Geometry: final body of the model. Coordinates: model frame, mm. Give positions to 0.01 mm unless a question says otherwise; leave off trailing zeros. Order: outer loops, then holes, each group sorted by start corner. A loop starts at its lowest first (then second) coordinate and runs counter-clockwise, first axis right, second up. Notation, with made-up numbers: (10, 38.25) -> (64, 38.25) arc R12 cw to (64, 60.25) -> close; hole circle Ø11 at (-7.5, 77.25). An arc over 180 degrees is marked (long way). Write item = value, one per line.
```python
from build123d import *

# Parameters (mm, degrees)
SKETCH1_R           = 4.7625
SKETCH1_W           = 1.5875
SKETCH1_H           = 0.79375
BOSS_EXTRUDE1_DEPTH = 25.4


with BuildPart() as part:
    # Sketch1 → Boss-Extrude1 (new body)
    with BuildSketch(Plane.XY):
        with Locations((-1.639930211, 2.216369181)):
            Circle(SKETCH1_R)
        with Locations((-1.639930211, 7.309385865)):
            Rectangle(SKETCH1_W, SKETCH1_H)
    extrude(amount=BOSS_EXTRUDE1_DEPTH)


solid = part.part
```
1) First-contact query: P1, Ø1.5, axis at y = 0, z = 20.5, coming from the -X side; P2, Ø4, axis at y = 6, z = 5.5, coming from the -X side. Flat tips, straight axial feed; report the tip coordinate or a pass-through.
Check sheet entries:
P1 = -6.17
P2 = -6.06
2) Section query C-C (y = -1.5). Output: boundary loops of the cut face in (x, z), plus the area to 3 significant figures.
Check sheet entries:
outline = (-4.62, 0) -> (1.34, 0) -> (1.34, 25.4) -> (-4.62, 25.4) -> close
area = 151 mm²
3) Line query: line 1 (X direction, y = 2, z = 7.5); line 2 (Y direction, x = -1.75, z = 15.25); line 3 (X direction, y = 7, z = 14.25). Output: solid intervals per line, ascending. Write a range as from..to.
Check sheet entries:
line_1 = -6.4..3.12
line_2 = -2.54..7.71
line_3 = -2.43..-0.85
4) Section query B-B (x = 2). Output: boundary loops of the cut face in (y, z), plus the area to 3 significant figures.
Check sheet entries:
outline = (-0.85, 0) -> (5.29, 0) -> (5.29, 25.4) -> (-0.85, 25.4) -> close
area = 156 mm²
